Can you work these out from the model? Positions are in its coordinate system, mm. A direction names the side the tool comes from. Coordinates: 2 decimals unless noted, no trailing zeros. Order: outer loops, then holes, each group sorted by start corner. A loop starts at its lowest first (then second) coordinate and runs counter-clockwise, first axis right, second up. Notation, with made-up numbers: (-19, 46) -> (18, 46) arc R26 cw to (18, 83) -> close; hole circle Ø10 at (7.25, 3.25). An arc over 180 degrees is marked (long way). Answer in a Markdown table with one row per item.
```python
from build123d import *

# Parameters (mm, degrees)
SKETCH1_W           = 126
SKETCH1_H           = 126
BOSS_EXTRUDE1_DEPTH = 5
SKETCH3_R           = 12.5
BOSS_EXTRUDE2_DEPTH = 7.5
SKETCH4_R           = 3.45
CUT_EXTRUDE1_DEPTH  = 11.5
SKETCH6_R           = 3
CUT_EXTRUDE2_DEPTH  = 179.628805068
CHAMFER1_SIZE       = 10
CHAMFER1_SIZE_2     = 7.26542528
SKETCH7_R           = 2.75
CUT_EXTRUDE3_DEPTH  = 179.348675353
CUT_EXTRUDE4_DEPTH  = 179.348675353


with BuildPart() as part:
    # Sketch1 → Boss-Extrude1 (new body)
    with BuildSketch(Plane(origin=(0, 0, 0), x_dir=(1, 0, 0), z_dir=(0, 1, 0))):
        with Locations((63, 63)):
            Rectangle(SKETCH1_W, SKETCH1_H)
    extrude(amount=BOSS_EXTRUDE1_DEPTH)

    # Sketch3 → Boss-Extrude2 (add)
    with BuildSketch(Plane(origin=(0, 5, 0), x_dir=(1, 0, 0), z_dir=(0, 1, 0))):
        with Locations(Location((108.6, 108.6, 0), (0, 0, 90))):
            Circle(SKETCH3_R)
    extrude(amount=BOSS_EXTRUDE2_DEPTH)

    # Sketch4 → Cut-Extrude1 (cut)
    with BuildSketch(Plane.XZ):
        with Locations(Location((108.6, -108.6, 0), (0, 0, 270))):
            Circle(SKETCH4_R)
    extrude(amount=-CUT_EXTRUDE1_DEPTH, mode=Mode.SUBTRACT)

    # Sketch6 → Cut-Extrude2 (cut, through all)
    with BuildSketch(Plane(origin=(0, 12.5, 0), x_dir=(1, 0, 0), z_dir=(0, 1, 0))):
        with Locations(Location((108.6, 108.6, 0), (0, 0, 270))):
            Circle(SKETCH6_R)
    extrude(amount=-CUT_EXTRUDE2_DEPTH, mode=Mode.SUBTRACT)

    # Chamfer1
    # the kernel refuses this chamfer: 10, 7.26542528 mm, written as the material it takes off along each edge
    with BuildSketch(Plane(origin=(108.6, 12.5, -108.6), x_dir=(0, 0, -1), z_dir=(1, 0, 0))) as chamfer1_piece_1_section:
        Polygon((12.5, -CHAMFER1_SIZE), (12.5 - CHAMFER1_SIZE_2, 0), (12.5, 0), align=None)
    chamfer1_piece_1 = revolve(axis=Axis((108.6, 12.5, -108.6), (0, 1, 0)), mode=Mode.PRIVATE)
    chamfer1_piece_1 = split(chamfer1_piece_1, bisect_by=Plane(origin=(108.6, 5, -108.6), z_dir=(0, 1, 0)), keep=Keep.TOP, mode=Mode.PRIVATE)
    add(chamfer1_piece_1, mode=Mode.SUBTRACT)

    # Sketch7 → Cut-Extrude3 (cut, through all)
    with BuildSketch(Plane(origin=(0, 5, 0), x_dir=(1, 0, 0), z_dir=(0, 1, 0))):
        with Locations(Location((55.5, 63, 0), (0, 0, 270))):
            Circle(SKETCH7_R)
        with Locations(Location((70.5, 63, 0), (0, 0, 270))):
            Circle(SKETCH7_R)
        with Locations(Location((40.5, 63, 0), (0, 0, 270))):
            Circle(SKETCH7_R)
        with Locations(Location((85.5, 63, 0), (0, 0, 270))):
            Circle(SKETCH7_R)
        with Locations(Location((25.5, 63, 0), (0, 0, 270))):
            Circle(SKETCH7_R)
        with Locations(Location((100.5, 63, 0), (0, 0, 270))):
            Circle(SKETCH7_R)
        with Locations(Location((25.5, 48, 0), (0, 0, 270))):
            Circle(SKETCH7_R)
        with Locations(Location((40.5, 48, 0), (0, 0, 270))):
            Circle(SKETCH7_R)
        with Locations(Location((55.5, 48, 0), (0, 0, 270))):
            Circle(SKETCH7_R)
        with Locations(Location((70.5, 48, 0), (0, 0, 270))):
            Circle(SKETCH7_R)
        with Locations(Location((85.5, 48, 0), (0, 0, 270))):
            Circle(SKETCH7_R)
        with Locations(Location((100.5, 48, 0), (0, 0, 270))):
            Circle(SKETCH7_R)
        with Locations(Location((25.5, 33, 0), (0, 0, 270))):
            Circle(SKETCH7_R)
        with Locations(Location((40.5, 33, 0), (0, 0, 270))):
            Circle(SKETCH7_R)
        with Locations(Location((55.5, 33, 0), (0, 0, 270))):
            Circle(SKETCH7_R)
        with Locations(Location((70.5, 33, 0), (0, 0, 270))):
            Circle(SKETCH7_R)
        with Locations(Location((85.5, 33, 0), (0, 0, 270))):
            Circle(SKETCH7_R)
        with Locations(Location((100.5, 33, 0), (0, 0, 270))):
            Circle(SKETCH7_R)
        with Locations(Location((25.5, 18, 0), (0, 0, 270))):
            Circle(SKETCH7_R)
        with Locations(Location((40.5, 18, 0), (0, 0, 270))):
            Circle(SKETCH7_R)
        with Locations(Location((55.5, 18, 0), (0, 0, 270))):
            Circle(SKETCH7_R)
        with Locations(Location((70.5, 18, 0), (0, 0, 270))):
            Circle(SKETCH7_R)
        with Locations(Location((85.5, 18, 0), (0, 0, 270))):
            Circle(SKETCH7_R)
        with Locations(Location((100.5, 18, 0), (0, 0, 270))):
            Circle(SKETCH7_R)
        with Locations(Location((25.5, 78, 0), (0, 0, 270))):
            Circle(SKETCH7_R)
        with Locations(Location((40.5, 78, 0), (0, 0, 270))):
            Circle(SKETCH7_R)
        with Locations(Location((55.5, 78, 0), (0, 0, 270))):
            Circle(SKETCH7_R)
        with Locations(Location((70.5, 78, 0), (0, 0, 270))):
            Circle(SKETCH7_R)
        with Locations(Location((85.5, 78, 0), (0, 0, 270))):
            Circle(SKETCH7_R)
        with Locations(Location((100.5, 78, 0), (0, 0, 270))):
            Circle(SKETCH7_R)
        with Locations(Location((25.5, 93, 0), (0, 0, 270))):
            Circle(SKETCH7_R)
        with Locations(Location((40.5, 93, 0), (0, 0, 270))):
            Circle(SKETCH7_R)
        with Locations(Location((55.5, 93, 0), (0, 0, 270))):
            Circle(SKETCH7_R)
        with Locations(Location((70.5, 93, 0), (0, 0, 270))):
            Circle(SKETCH7_R)
        with Locations(Location((85.5, 93, 0), (0, 0, 270))):
            Circle(SKETCH7_R)
        with Locations(Location((100.5, 93, 0), (0, 0, 270))):
            Circle(SKETCH7_R)
    extrude(amount=-CUT_EXTRUDE3_DEPTH, mode=Mode.SUBTRACT)

    # Sketch8 → Cut-Extrude4 (cut, through all)
    with BuildSketch(Plane(origin=(0, 5, 0), x_dir=(1, 0, 0), z_dir=(0, 1, 0))):
        Polygon((70.5, 100.75), (63, 108.375), (55.5, 100.75), align=None)
        Polygon((108.25, 63), (115.875, 55.5), (108.25, 48), align=None)
        Polygon((55.5, 10.25), (63, 2.625), (70.5, 10.25), align=None)
        Polygon((17.75, 63), (17.75, 48), (10.125, 55.5), align=None)
    extrude(amount=-CUT_EXTRUDE4_DEPTH, mode=Mode.SUBTRACT)


solid = part.part
```
(1) Suppose I cut it at A-A (x = 85.5). Please give me the cut outline in (y, z), and give its area (3 significant figures).
Response values:
| item | result |
|---|---|
| outline | (0, -126) -> (5, -126) -> (5, -95.75) -> (0, -95.75) -> close; (0, -90.25) -> (5, -90.25) -> (5, -80.75) -> (0, -80.75) -> close; (0, -75.25) -> (5, -75.25) -> (5, -65.75) -> (0, -65.75) -> close; (0, -60.25) -> (5, -60.25) -> (5, -50.75) -> (0, -50.75) -> close; (0, -45.25) -> (5, -45.25) -> (5, -35.75) -> (0, -35.75) -> close; (0, -30.25) -> (5, -30.25) -> (5, -20.75) -> (0, -20.75) -> close; (0, -15.25) -> (5, -15.25) -> (5, 0) -> (0, 0) -> close |
| area | 465 mm2 |
(2) On a 3-axis mill with a long thin cutter (end or side, diameter ignored), from which of +Z, -Z, +X, -X, +Y, -Y can I reach the whole of each face in a straight line? I mean faces 1 (the flat face through (62, 2, -126)), 2 (the flat face through (59.2, 2.54, -6.49)). Say none if no direction works.
Response values:
| item | result |
|---|---|
| face 1 | -Z, +X, -X, +Y, -Y |
| face 2 | +Y, -Y |
(3) Will this pin go through, and if not, where does the flat tip stop? pin 1 Ø4 at (x, z) = (63, -51.5) entering from +Y.
Response values:
| item | result |
|---|---|
| pin 1 | y = 5 |
(4) I need wall thicknesses on line 1 (X direction, y = 4.25, z = -108.6); line 2 (Y direction, x = 24.5, z = -13); line 3 (X direction, y = 9.75, z = -106.5). Which ranges of each line are inside material? Lowest first, please. Write a range as [from, to].
Response values:
| item | result |
|---|---|
| line 1 | [0, 105.15], [112.05, 126] |
| line 2 | [0, 5] |
| line 3 | [101.68, 105.86], [111.34, 115.52] |
(5) Suppose I cut it at C-C (y = 2.75). Count the separate pieces of the cut face and the enclosed holes in it, and give its area (3 significant figures).
Response values:
| item | result |
|---|---|
| separate pieces | 1 |
| enclosed holes | 41 |
| area | 14,800 mm2 |
(6) We'd pull the mould along Y, two halves only. Please class faces 3 (the flat face through (62, 0, -64)), 4 (the cylindrical face through (42.359, 2.535, -50.027)): +Y half, -Y half, draft (parallel to the pull), parting line (faces both ways), or undercut.
Response values:
| item | result |
|---|---|
| face 3 | -Y half |
| face 4 | draft |
(7) Suppose I cut it at B-B (z = -18). Please give me the cut outline in (x, y), and give its area (3 significant figures).
Response values:
| item | result |
|---|---|
| outline | (0, 0) -> (22.75, 0) -> (22.75, 5) -> (0, 5) -> close; (28.25, 0) -> (37.75, 0) -> (37.75, 5) -> (28.25, 5) -> close; (43.25, 0) -> (52.75, 0) -> (52.75, 5) -> (43.25, 5) -> close; (58.25, 0) -> (67.75, 0) -> (67.75, 5) -> (58.25, 5) -> close; (73.25, 0) -> (82.75, 0) -> (82.75, 5) -> (73.25, 5) -> close; (88.25, 0) -> (97.75, 0) -> (97.75, 5) -> (88.25, 5) -> close; (103.25, 0) -> (126, 0) -> (126, 5) -> (103.25, 5) -> close |
| area | 465 mm2 |
